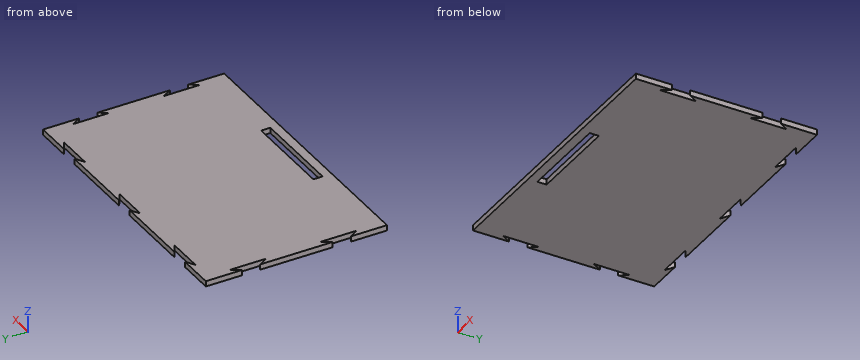
```python
from build123d import *

# Parameters (mm, degrees)
ESQUISSE1_W             = 156
ESQUISSE1_H             = 100
BOSS_EXTRU_1_DEPTH      = 3
ENL_V_MAT_EXTRU_1_DEPTH = 3
ENL_V_MAT_EXTRU_3_DEPTH = 3
ENL_V_MAT_EXTRU_4_DEPTH = 3
ESQUISSE6_W             = 50.1
ESQUISSE6_H             = 5.1
ENL_V_MAT_EXTRU_5_DEPTH = 3


with BuildPart() as part:
    # Esquisse1 → Boss.-Extru.1 (new body)
    with BuildSketch(Plane.XY):
        Rectangle(ESQUISSE1_W, ESQUISSE1_H)
    extrude(amount=BOSS_EXTRU_1_DEPTH)

    # Esquisse2 → Enlèv. mat.-Extru.1 (cut)
    with BuildSketch(Plane(origin=(0, 0, 0), x_dir=(-1, 0, 0), z_dir=(0, 0, -1))):
        Polygon((-58, 50), (-63, 47), (-43, 47), (-48, 50), align=None)
        Polygon((-10, 47), (-5, 50), (5, 50), (10, 47), align=None)
        Polygon((48, 50), (43, 47), (63, 47), (58, 50), align=None)
    extrude(amount=-ENL_V_MAT_EXTRU_1_DEPTH, mode=Mode.SUBTRACT)

    # Esquisse4 → Enlèv. mat.-Extru.3 (cut)
    with BuildSketch(Plane(origin=(0, 0, 0), x_dir=(-1, 0, 0), z_dir=(0, 0, -1))):
        Polygon((-78, 30), (-75, 35), (-75, 15), (-78, 20), align=None)
        Polygon((-78, -20), (-75, -15), (-75, -35), (-78, -30), align=None)
    extrude(amount=-ENL_V_MAT_EXTRU_3_DEPTH, mode=Mode.SUBTRACT)

    # Esquisse5 → Enlèv. mat.-Extru.4 (cut)
    with BuildSketch(Plane(origin=(0, 0, 0), x_dir=(-1, 0, 0), z_dir=(0, 0, -1))):
        Polygon((78, 30), (75, 35), (75, 15), (78, 20), align=None)
        Polygon((78, -20), (75, -15), (75, -35), (78, -30), align=None)
    extrude(amount=-ENL_V_MAT_EXTRU_4_DEPTH, mode=Mode.SUBTRACT)

    # Esquisse6 → Enlèv. mat.-Extru.5 (cut)
    with BuildSketch(Plane(origin=(0, 0, 0), x_dir=(-1, 0, 0), z_dir=(0, 0, -1))):
        with Locations((-0.05, -42.45)):
            Rectangle(ESQUISSE6_W, ESQUISSE6_H)
    extrude(amount=-ENL_V_MAT_EXTRU_5_DEPTH, mode=Mode.SUBTRACT)


solid = part.part
```
The listing builds one solid part. Answer for the finished solid, in the listing's coordinates (mm). Round coordinates to 2 decimals unless told otherwise and drop trailing zeros. Loops run counter-clockwise (first coordinate to the right, second up) from the corner with the lowest first, then second, coordinate; pieces in that order, holes last.
Q1. Section A-A, the plane x = -7.5 is taken. Determine the outline of the cut face in (y, z).
Q2. Find the intervals of material crossed by line 1 (X direction, y = -18.5, z = 1.1); line 2 (Y direction, x = 22.5, z = 2.15); line 3 (X direction, y = -23.5, z = 0.5), in increasing order.
Q3. Section B-B, the plane x = 23 is taken. Determine the outline of the cut face in (y, z), then the cut area to 3 significant figures.
Q4. Given pin 1 Ø1.5 at (y, z) = (-29.5, 1.5) entering from -X; pin 2 Ø0.9 at (y, z) = (24.5, 1) entering from -X; pin 3 Ø0.9 at (x, z) = (-4, 2) entering from +Y, each flat-ended and moving along its own axis, determine where each tip first touches the part or whether it passes through.
Q5. Section C-C, the plane y = -23.5 is taken. Determine the outline of the cut face in (x, z).
Q6. Section D-D, the plane x = -56.5 is taken. Determine the outline of the cut face in (y, z).
Completed:
1. outline: (-50, 0) - (-45, 0) - (-45, 3) - (-50, 3) - close; (-39.9, 0) - (47, 0) - (47, 3) - (-39.9, 3) - close; (48.5, 0) - (50, 0) - (50, 3) - (48.5, 3) - close
2. line 1: x = -78 to -77.1, -75 to 75, 77.1 to 78
2. line 2: y = -50 to -45, -39.9 to 50
2. line 3: x = -75 to 75
3. outline: (-50, 0) - (-45, 0) - (-45, 3) - (-50, 3) - close; (-39.9, 0) - (50, 0) - (50, 3) - (-39.9, 3) - close
3. area: 285 mm2
4. pin 1: stops at x = -78
4. pin 2: stops at x = -75
4. pin 3: stops at y = 47
5. outline: (-75, 0) - (75, 0) - (75, 3) - (-75, 3) - close
6. outline: (-50, 0) - (47, 0) - (47, 3) - (-50, 3) - close
